Could you check a few things on this model? Use its own coordinates, in mm. Face numbers are marked on the shaded views. A direction names the side the tool comes from. Give positions to 0.01 mm unless a question says otherwise; leave off trailing zeros. Loops run counter-clockwise (first coordinate to the right, second up) from the corner with the lowest first, then second, coordinate; pieces in that order, holes last. Notation, with made-up numbers: (7, -38.75) - (59, -38.75) arc R13 ccw to (59, -21.75) - close; hole circle Ø6 at (59.25, 64). An arc over 180 degrees is marked (long way). One line per item, written item: value. Start each with the question number.
Q1. If I drill on line 1 (Z direction, x = -12, y = 1); line 2 (Z direction, x = -0.5, y = 13); line 3 (X direction, y = 10, z = 5.5), over which ranges is the centre line in solid material (lowest first)? Write a range as from..to.
Q2. I'm going to push flat-ended pins straight in: P1, Ø1, axis at x = -2, z = 13, coming from the +Y side; P2, Ø4, axis at x = 9.89, y = 13.83, coming from the +Z side; P3, Ø1.5, axis at x = -16, y = 16, coming from the -Z side. Where does each tip first touch, or does it pass through?
Q3. If we mould it in two halves opening along X, with no side actions, what happens to the marked faces 4, 5 and 6? For each: released by +X, released by -X, zero draft, split by the parting line, or undercut.
Q4. For the marked faces 1, 2 and 3, which set-ups out of +Z, -Z, +X, -X, +Y, -Y let a thin tool reach every point of the face, with its end or its side?
Q5. I want a section at C-C (z = 77.5). Please give me the cut outline in (x, y).
Q6. I want a section at B-B (z = 15.5). Please give me the cut outline in (x, y).
Q7. I want a section at A-A (z = 53). Please give me the cut outline in (x, y).
```python
from build123d import *

# Parameters (mm, degrees)
SKETCH1_R           = 21
BOSS_EXTRUDE1_DEPTH = 66.5
SKETCH2_R           = 8.5
BOSS_EXTRUDE2_DEPTH = 2
BOSS_EXTRUDE3_START = 8
SKETCH4_R           = 2.5
BOSS_EXTRUDE3_DEPTH = 92.5
CHAMFER1_SIZE       = 0.15
SKETCH5_R           = 1.5
CUT_EXTRUDE1_DEPTH  = 5
SKETCH7_W           = 3
SKETCH7_H           = 5
CUT_EXTRUDE2_DEPTH  = 0.5
CUT_EXTRUDE3_DEPTH  = 5
BOSS_EXTRUDE4_START = -30
SKETCH9_R           = 22
BOSS_EXTRUDE4_DEPTH = 30
CUT_EXTRUDE5_START  = -2
SKETCH10_R          = 20
SKETCH10_R_2        = 12.5
CUT_EXTRUDE5_DEPTH  = 59.5
SKETCH12_R          = 5
SKETCH12_R_2        = 2.6
BOSS_EXTRUDE5_DEPTH = 4
CHAMFER2_SIZE       = 2
SKETCH14_R          = 20
SKETCH14_R_2        = 14
CUT_EXTRUDE6_DEPTH  = 0.3
SKETCH15_R          = 7
SKETCH15_R_2        = 2.6
CUT_EXTRUDE7_DEPTH  = 0.2
SKETCH16_R          = 5.25
SKETCH16_R_2        = 5
CUT_EXTRUDE8_DEPTH  = 5
SKETCH17_R          = 1.25
CUT_EXTRUDE9_DEPTH  = 0.3
CUT_EXTRUDE12_DEPTH = 1.5
CUT_EXTRUDE13_START = -1
SKETCH20_R          = 20
SKETCH20_R_2        = 2.5
CUT_EXTRUDE13_DEPTH = 1
FILLET1_R           = 2


with BuildPart() as part:
    # Sketch1 → Boss-Extrude1 (new body)
    with BuildSketch(Plane.XY):
        Circle(SKETCH1_R)
    extrude(amount=BOSS_EXTRUDE1_DEPTH)

    # Sketch2 → Boss-Extrude2 (add)
    with BuildSketch(Plane.XY.offset(66.5)):
        Circle(SKETCH2_R)
    extrude(amount=BOSS_EXTRUDE2_DEPTH)

    # Sketch4 → Boss-Extrude3 (add)
    with BuildSketch(Plane(origin=(0, 0, 0), x_dir=(-1, 0, 0), z_dir=(0, 0, -1)).offset(BOSS_EXTRUDE3_START)):
        Circle(SKETCH4_R)
    extrude(amount=-BOSS_EXTRUDE3_DEPTH)

    # Chamfer1
    chamfer1_edges = [part.edges().sort_by_distance(p)[0] for p in [
        (2.5, 0, 84.5),
        (2.5, 0, -8),
    ]]
    chamfer(chamfer1_edges, length=CHAMFER1_SIZE)

    # Sketch5 → Cut-Extrude1 (cut)
    with BuildSketch(Plane.XY.offset(66.5)):
        with Locations((0, 14.5)):
            Circle(SKETCH5_R)
        with Locations((14.5, 0)):
            Circle(SKETCH5_R)
        with Locations((0, -14.5)):
            Circle(SKETCH5_R)
        with Locations((-14.5, 0)):
            Circle(SKETCH5_R)
    extrude(amount=-CUT_EXTRUDE1_DEPTH, mode=Mode.SUBTRACT)

    # Sketch7 → Cut-Extrude2 (cut)
    with BuildSketch(Plane(origin=(0, 0, 0), x_dir=(-1, 0, 0), z_dir=(0, 0, -1))):
        with Locations((19.5, 0)):
            Rectangle(SKETCH7_W, SKETCH7_H)
        with Locations((-19.5, 0)):
            Rectangle(SKETCH7_W, SKETCH7_H)
    extrude(amount=-CUT_EXTRUDE2_DEPTH, mode=Mode.SUBTRACT)

    # Sketch8 → Cut-Extrude3 (cut)
    with BuildSketch(Plane.XY.offset(66.5)):
        with BuildLine():
            Line((6.761892188, 14.500924593), (5.494037403, 11.782001231))
            ThreePointArc((5.494037403, 11.782001231), (9.192388155, 9.192388155), (11.782001231, 5.494037403))
            Line((11.782001231, 5.494037403), (14.500924593, 6.761892188))
            ThreePointArc((14.500924593, 6.761892188), (11.313708499, 11.313708499), (6.761892188, 14.500924593))
        make_face()
        with BuildLine():
            Line((5.494037403, -11.782001231), (6.761892188, -14.500924593))
            ThreePointArc((6.761892188, -14.500924593), (11.313708499, -11.313708499), (14.500924593, -6.761892188))
            Line((14.500924593, -6.761892188), (11.782001231, -5.494037403))
            ThreePointArc((11.782001231, -5.494037403), (9.192388155, -9.192388155), (5.494037403, -11.782001231))
        make_face()
        with BuildLine():
            Line((-11.782001231, -5.494037403), (-14.500924593, -6.761892188))
            ThreePointArc((-14.500924593, -6.761892188), (-11.313708499, -11.313708499), (-6.761892188, -14.500924593))
            Line((-6.761892188, -14.500924593), (-5.494037403, -11.782001231))
            ThreePointArc((-5.494037403, -11.782001231), (-9.192388155, -9.192388155), (-11.782001231, -5.494037403))
        make_face()
        with BuildLine():
            Line((-5.494037403, 11.782001231), (-6.761892188, 14.500924593))
            ThreePointArc((-6.761892188, 14.500924593), (-11.313708499, 11.313708499), (-14.500924593, 6.761892188))
            Line((-14.500924593, 6.761892188), (-11.782001231, 5.494037403))
            ThreePointArc((-11.782001231, 5.494037403), (-9.192388155, 9.192388155), (-5.494037403, 11.782001231))
        make_face()
    extrude(amount=-CUT_EXTRUDE3_DEPTH, mode=Mode.SUBTRACT)

    # Sketch9 → Boss-Extrude4 (add)
    with BuildSketch(Plane(origin=(0, 0, 0), x_dir=(-1, 0, 0), z_dir=(0, 0, -1)).offset(BOSS_EXTRUDE4_START)):
        Circle(SKETCH9_R)
    extrude(amount=-BOSS_EXTRUDE4_DEPTH)

    # Sketch10 → Cut-Extrude5 (cut)
    with BuildSketch(Plane(origin=(0, 0, 0), x_dir=(-1, 0, 0), z_dir=(0, 0, -1)).offset(CUT_EXTRUDE5_START)):
        Circle(SKETCH10_R)
        Circle(SKETCH10_R_2, mode=Mode.SUBTRACT)
    extrude(amount=-CUT_EXTRUDE5_DEPTH, mode=Mode.SUBTRACT)

    # Sketch12 → Boss-Extrude5 (add)
    with BuildSketch(Plane(origin=(0, 0, 0), x_dir=(-1, 0, 0), z_dir=(0, 0, -1))):
        with Locations(Location((0, 0, 0), (0, 0, 180))):
            Circle(SKETCH12_R)
        Circle(SKETCH12_R_2, mode=Mode.SUBTRACT)
    extrude(amount=BOSS_EXTRUDE5_DEPTH)

    # Chamfer2
    chamfer2_edges = [part.edges().sort_by_distance(p)[0] for p in [
        (-5, 0, -4),
    ]]
    chamfer(chamfer2_edges, length=CHAMFER2_SIZE)

    # Sketch14 → Cut-Extrude6 (cut)
    with BuildSketch(Plane(origin=(0, 0, 0), x_dir=(-1, 0, 0), z_dir=(0, 0, -1))):
        Circle(SKETCH14_R)
        Circle(SKETCH14_R_2, mode=Mode.SUBTRACT)
    extrude(amount=-CUT_EXTRUDE6_DEPTH, mode=Mode.SUBTRACT)

    # Sketch15 → Cut-Extrude7 (cut)
    with BuildSketch(Plane.XY.offset(68.5)):
        Circle(SKETCH15_R)
        with Locations(Location((0, 0, 0), (0, 0, 180))):
            Circle(SKETCH15_R_2, mode=Mode.SUBTRACT)
    extrude(amount=-CUT_EXTRUDE7_DEPTH, mode=Mode.SUBTRACT)

    # Sketch16 → Cut-Extrude8 (cut)
    with BuildSketch(Plane.XY.offset(68.3)):
        Circle(SKETCH16_R)
        Circle(SKETCH16_R_2, mode=Mode.SUBTRACT)
    extrude(amount=-CUT_EXTRUDE8_DEPTH, mode=Mode.SUBTRACT)

    # Sketch17 → Cut-Extrude9 (cut)
    with BuildSketch(Plane(origin=(0, 0, 0.3), x_dir=(-1, 0, 0), z_dir=(0, 0, -1))):
        with Locations((13.826532207, 9.893378466)):
            Circle(SKETCH17_R)
        with Locations(Location((9.893378466, 13.826532207, 0), (0, 0, 180))):
            Circle(SKETCH17_R)
        with Locations(Location((13.826532207, -9.893378466, 0), (0, 0, 180))):
            Circle(SKETCH17_R)
        with Locations((9.893378466, -13.826532207)):
            Circle(SKETCH17_R)
        with Locations(Location((-9.893378466, -13.826532207, 0), (0, 0, 180))):
            Circle(SKETCH17_R)
        with Locations((-13.826532207, -9.893378466)):
            Circle(SKETCH17_R)
        with Locations(Location((-13.826532207, 9.893378466, 0), (0, 0, 180))):
            Circle(SKETCH17_R)
        with Locations((-9.893378466, 13.826532207)):
            Circle(SKETCH17_R)
    extrude(amount=-CUT_EXTRUDE9_DEPTH, mode=Mode.SUBTRACT)

    # Sketch19 → Cut-Extrude12 (cut)
    with BuildSketch(Plane(origin=(0, 0, 0), x_dir=(-1, 0, 0), z_dir=(0, 0, -1))):
        with BuildLine():
            ThreePointArc((-7.987387277, -2.907171218), (-6.01040764, -6.01040764), (-2.907171218, -7.987387277))
            Line((-2.907171218, -7.987387277), (-4.275251792, -11.74615776))
            ThreePointArc((-4.275251792, -11.74615776), (-8.838834765, -8.838834765), (-11.74615776, -4.275251792))
            Line((-11.74615776, -4.275251792), (-7.987387277, -2.907171218))
        make_face()
        with BuildLine():
            ThreePointArc((7.987387277, 2.907171218), (6.01040764, 6.01040764), (2.907171218, 7.987387277))
            Line((2.907171218, 7.987387277), (4.275251792, 11.74615776))
            ThreePointArc((4.275251792, 11.74615776), (8.838834765, 8.838834765), (11.74615776, 4.275251792))
            Line((11.74615776, 4.275251792), (7.987387277, 2.907171218))
        make_face()
        with BuildLine():
            ThreePointArc((2.907171218, -7.987387277), (6.01040764, -6.01040764), (7.987387277, -2.907171218))
            Line((7.987387277, -2.907171218), (11.74615776, -4.275251792))
            ThreePointArc((11.74615776, -4.275251792), (8.838834765, -8.838834765), (4.275251792, -11.74615776))
            Line((4.275251792, -11.74615776), (2.907171218, -7.987387277))
        make_face()
        with BuildLine():
            ThreePointArc((-2.907171218, 7.987387277), (-6.01040764, 6.01040764), (-7.987387277, 2.907171218))
            Line((-7.987387277, 2.907171218), (-11.74615776, 4.275251792))
            ThreePointArc((-11.74615776, 4.275251792), (-8.838834765, 8.838834765), (-4.275251792, 11.74615776))
            Line((-4.275251792, 11.74615776), (-2.907171218, 7.987387277))
        make_face()
    extrude(amount=-CUT_EXTRUDE12_DEPTH, mode=Mode.SUBTRACT)

    # Sketch20 → Cut-Extrude13 (cut)
    with BuildSketch(Plane(origin=(0, 0, 0), x_dir=(-1, 0, 0), z_dir=(0, 0, -1)).offset(CUT_EXTRUDE13_START)):
        Circle(SKETCH20_R)
        Circle(SKETCH20_R_2, mode=Mode.SUBTRACT)
    extrude(amount=-CUT_EXTRUDE13_DEPTH, mode=Mode.SUBTRACT)

    # Fillet1
    fillet1_edges = [part.edges().sort_by_distance(p)[0] for p in [
        (2.907171218, -7.987387277, 0.5),
        (4.275251792, -11.74615776, 0.5),
        (-4.275251792, -11.74615776, 0.5),
        (-11.74615776, -4.275251792, 0.5),
        (-2.907171218, -7.987387277, 0.5),
        (11.74615776, -4.275251792, 0.5),
        (7.987387277, -2.907171218, 0.5),
        (-7.987387277, -2.907171218, 0.5),
        (-11.74615776, 4.275251792, 0.5),
        (-7.987387277, 2.907171218, 0.5),
        (7.987387277, 2.907171218, 0.5),
        (2.907171218, 7.987387277, 0.5),
        (4.275251792, 11.74615776, 0.5),
        (11.74615776, 4.275251792, 0.5),
        (-2.907171218, 7.987387277, 0.5),
        (-4.275251792, 11.74615776, 0.5),
    ]]
    fillet(fillet1_edges, radius=FILLET1_R - 0.0001)  # a hair under: the kernel refuses the full size


solid = part.part
```
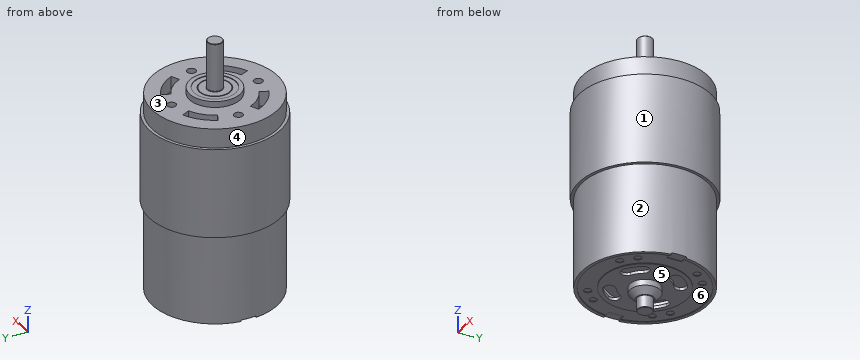
Worked answers:
1. line 1: z = 0..1, 2..66.5
1. line 2: z = 0..1, 61.5..66.5
1. line 3: x = -18.47..-17.32, -7.5..7.5, 17.32..18.47
2. P1: stops at y = 20.95
2. P2: stops at z = 66.5
2. P3: stops at z = 30
3. face 4: split by the parting line
3. face 5: zero draft
3. face 6: undercut
4. face 1: +Z, -Z
4. face 2: -Z
4. face 3: +Z
5. outline: circle Ø5 at (0, 0)
6. outline: circle Ø42 at (0, 0); circle Ø25 at (0, 0); hole circle Ø40 at (0, 0)
7. outline: circle Ø44 at (0, 0); circle Ø25 at (0, 0); hole circle Ø40 at (0, 0)
